from build123d import *

# Parameters (mm, degrees)
BOSS_EXTRUDE1_DEPTH = 5
SKETCH2_R           = 4
SKETCH2_R_2         = 1
CUT_EXTRUDE1_DEPTH  = 5
SKETCH3_R           = 5
BOSS_EXTRUDE3_DEPTH = 2
DRAFT3_ANGLE        = 30
SKETCH4_R           = 4
CUT_EXTRUDE2_DEPTH  = 2
SKETCH5_R           = 4
SKETCH5_R_2         = 2.700917016
BOSS_EXTRUDE4_DEPTH = 2
SKETCH6_R           = 4.5
SKETCH6_R_2         = 4
BOSS_EXTRUDE5_DEPTH = 1
DRAFT4_ANGLE        = 30


with BuildPart() as part:
    # Sketch1 → Boss-Extrude1 (new body)
    with BuildSketch(Plane(origin=(0, 0, 0), x_dir=(1, 0, 0), z_dir=(0, 1, 0))):
        with BuildLine():
            Line((-7.5, 0), (-5, 30))
            ThreePointArc((-5, 30), (0, 35), (5, 30))
            Line((5, 30), (7.5, 0))
            ThreePointArc((7.5, 0), (0, -7.5), (-7.5, 0))
        make_face()
    extrude(amount=BOSS_EXTRUDE1_DEPTH)

    # Sketch2 → Cut-Extrude1 (cut)
    with BuildSketch(Plane(origin=(0, 5, 0), x_dir=(1, 0, 0), z_dir=(0, 1, 0))):
        Circle(SKETCH2_R)
        with Locations((0, 30)):
            Circle(SKETCH2_R_2)
    extrude(amount=-CUT_EXTRUDE1_DEPTH, mode=Mode.SUBTRACT)

    # Sketch3 → Boss-Extrude3 (add)
    with BuildSketch(Plane.XZ):
        Circle(SKETCH3_R)
    extrude(amount=BOSS_EXTRUDE3_DEPTH)

    # Draft3
    draft3_faces = [part.faces().sort_by_distance(p)[0] for p in [
        (-5, -1, 0),
    ]]
    draft(draft3_faces, Plane(origin=(0, -2, 0), x_dir=(0, 0, -1), z_dir=(0, -1, 0)), DRAFT3_ANGLE)

    # Sketch4 → Cut-Extrude2 (cut)
    with BuildSketch(Plane(origin=(0, 0, 0), x_dir=(1, 0, 0), z_dir=(0, 1, 0))):
        Circle(SKETCH4_R)
    extrude(amount=-CUT_EXTRUDE2_DEPTH, mode=Mode.SUBTRACT)

    # Sketch5 → Boss-Extrude4 (add)
    with BuildSketch(Plane(origin=(0, 5, 0), x_dir=(1, 0, 0), z_dir=(0, 1, 0))):
        Circle(SKETCH5_R)
        Circle(SKETCH5_R_2, mode=Mode.SUBTRACT)
    extrude(amount=-BOSS_EXTRUDE4_DEPTH)

    # Sketch6 → Boss-Extrude5 (add)
    with BuildSketch(Plane(origin=(0, 5, 0), x_dir=(1, 0, 0), z_dir=(0, 1, 0))):
        Circle(SKETCH6_R)
        Circle(SKETCH6_R_2, mode=Mode.SUBTRACT)
    extrude(amount=BOSS_EXTRUDE5_DEPTH)

    # Draft4
    draft4_faces = [part.faces().sort_by_distance(p)[0] for p in [
        (-4.5, 5.5, 0),
    ]]
    draft(draft4_faces, Plane.ZX.offset(6), DRAFT4_ANGLE)


solid = part.part
Build history of the part. All positions in model axes, mm. A direction names the side the tool comes from. Coordinates: 2 decimals unless noted, no trailing zeros. Order: outer loops, then holes, each group sorted by start corner. A loop starts at its lowest first (then second) coordinate and runs counter-clockwise, first axis right, second up. Notation, with made-up numbers: M 74.5,39 L 89.5,39 A14 ccw 89.5,43 Z; hole C 8,49 d9. An arc over 180 degrees is marked long. One line per question, with ' | ' between items. Start each with the question number.
Q1. Saw through at B-B (y = 2.5). List the corners of the cut face in (x, z).
Q2. Flat gauge pins, fed straight in: pin 1 Ø1.5 at (x, z) = (0, -13.5) entering from -Y; pin 2 Ø9 at (x, z) = (0, 1) entering from -Y; pin 3 Ø6.5 at (x, z) = (0, 0) entering from +Y; pin 4 Ø7 at (x, z) = (0, 0) entering from -Y. Where does each tip first touch, or does it go through?
Q3. Probe L1, parallel to Z at x = 0, y = 4.4; L2, parallel to X at y = 1.65, z = -30; L3, parallel to Z at x = -0.5, y = 1.5. List the from-to ranges inside material, lowest first. Write a range as from..to.
Q4. Two-plate mould, pull along Z, no slides. Class faces 4 (the face through (0, 0, -19)), 5 (the face through (-0.867, 5.493, 3.905)), 6 (the face through (6.232, 2.465, -15.21)): +Z half, -Z half, draft (parallel to the pull), parting line (faces both ways), or undercut.
Q5. 3-axis set-ups, long thin cutter, end or side, ignore diameter. For faces 1 (the face through (-0.867, 0.535, 3.905)), 2 (the face through (-3, 6, 3)), 3 (the face through (3, 5, 1)): which of +Z, -Z, +X, -X, +Y, -Y reach the whole face in a straight line?
Q6. Saw through at C-C (y = -1). List the corners of the cut face in (x, z).
Q7. Saw through at D-D (z = -25). List the corners of the cut face in (x, y).
Q8. Saw through at A-A (x = 0). List the corners of the cut face in (y, z), then the cut area to 3 significant figures.
Check values:
1) outline: M -7.5,0 L -5,-30 A5 ccw 5,-30 L 7.5,0 A7.5 ccw Z; hole C 0,0 d8; hole C 0,-30 d2
2) pin 1: stops at y = 0 | pin 2: stops at y = -2 | pin 3: stops at y = 5 | pin 4: stops at y = 3
3) L1: z = -35..-31, -29..-2.7, 2.7..7.5 | L2: x = -5..-1, 1..5 | L3: z = -34.97..-30.87, -29.13..-3.97, 3.97..7.48
4) face 4: draft | face 5: undercut | face 6: -Z half
5) face 1: -Y | face 2: +Z, -Z, +X, -X, +Y | face 3: +Y
6) outline: C 0,0 d11.15; hole C 0,0 d8
7) outline: M -5.42,0 L 5.42,0 L 5.42,5 L -5.42,5 Z
8) outline: M -2,-5 L 0,-6.15 L 0,-29 L 5,-29 L 5,-5.08 L 6,-4.5 L 6,-4 L 5,-4 L 5,-2.7 L 3,-2.7 L 3,-4 L -2,-4 Z; M -2,4 L 3,4 L 3,2.7 L 5,2.7 L 5,4 L 6,4 L 6,4.5 L 5,5.08 L 5,7.5 L 0,7.5 L 0,6.15 L -2,5 Z; M 0,-35 L 5,-35 L 5,-31 L 0,-31 Z | area: 176 mm2
